Here's how the part is built. I have some questions about the finished solid (model axes, mm). Coordinates: 2 decimals unless noted, no trailing zeros. Write each loop counter-clockwise with the first axis right and the second up, starting at its lowest first coordinate (ties: lowest second). Pieces come first, ordered by that corner, then holes. Notation, with made-up numbers: (-26, -4) - (-19, -4) arc R31 cw to (-19, 30) - close; hole circle Ø8 at (55, -2.75). An arc over 180 degrees is marked (long way). Answer in a Markdown table with one row per item. Add a question column.
Item 1: Imagine slicing it at C-C (x = -20). Please give me the cut outline in (y, z).
Item 2: Imagine slicing it at A-A (y = -22.2). Please give me the cut outline in (x, z), plus the area to 3 significant figures.
Item 3: If I drill on probe 1 along Y at (x, z) = (-20, -6); probe 2 along X at (y, z) = (22.2, -6.25); probe 3 along Y at (x, z) = (-13, -1.75), over which ranges is the centre line in solid material (lowest first)? Write a range as from..to.
Item 4: Imagine slicing it at D-D (z = -9). Please give me the cut outline in (x, y).
Item 5: Imagine slicing it at B-B (x = 13). Please give me the cut outline in (y, z), plus the area to 3 significant figures.
Item 6: I'm going to push a flat-ended pin straight in: pin 1 (4 mm diameter, centred on x = 13, y = 0, fed in from -Z). Where does the tip first touch, or does it pass through?
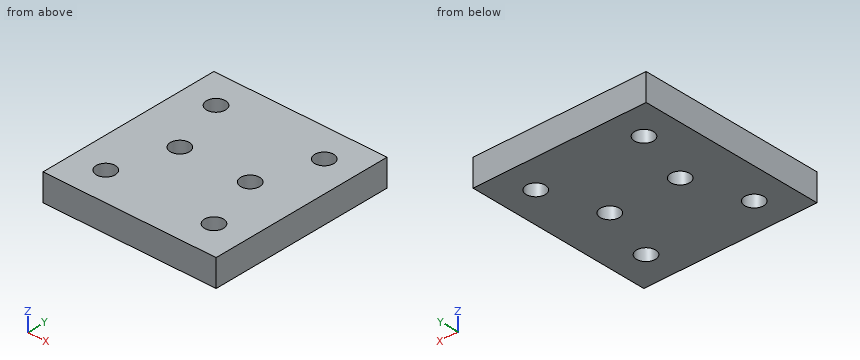
Solid Edge part; units mm, degrees
sketch "Sketch1" plane through (0, 0, 0) normal (0, 0, 1) x (1, 0, 0)
  line L0 (32, -10) -> (32, 10)
  line L1 (32, 10) -> (32, 34.4)
  line L2 (32, 34.4) -> (-32, 34.4)
  line L3 (-32, 34.4) -> (-32, 10)
  line L4 (-32, 10) -> (-32, -10)
  line L5 (-32, -10) -> (-32, -34.4)
  line L6 (-32, -34.4) -> (32, -34.4)
  line L7 (32, -34.4) -> (32, -10)
extrude "Protrusion1" add sketch "Sketch1" against normal blind 10
hole "Hole_1" at (20, -22.2, 0) direction (0, 0, -1) diameter 7 end up to next
mirror "Mirror1" about plane through (0, 0, 0) normal (1, 0, 0) of "Hole_1"
mirror "Mirror2" about plane through (0, 0, 0) normal (0, -1, 0) of "Mirror1", "Hole_1"
hole "Hole_4" at (13, 0, 0) direction (0, 0, -1) diameter 7 end up to next
hole "Hole2" at (-13, 0, 0) direction (0, 0, -1) diameter 7 end up to next
Here are the results:
| question | item | result |
|---|---|---|
| 1 | outline | (-34.4, -10) - (-25.7, -10) - (-25.7, 0) - (-34.4, 0) - close; (-18.7, -10) - (18.7, -10) - (18.7, 0) - (-18.7, 0) - close; (25.7, -10) - (34.4, -10) - (34.4, 0) - (25.7, 0) - close |
| 2 | outline | (-32, -10) - (-23.5, -10) - (-23.5, 0) - (-32, 0) - close; (-16.5, -10) - (16.5, -10) - (16.5, 0) - (-16.5, 0) - close; (23.5, -10) - (32, -10) - (32, 0) - (23.5, 0) - close |
| 2 | area | 500 mm2 |
| 3 | probe 1 | y = -34.4..-25.7, -18.7..18.7, 25.7..34.4 |
| 3 | probe 2 | x = -32..-23.5, -16.5..16.5, 23.5..32 |
| 3 | probe 3 | y = -34.4..-3.5, 3.5..34.4 |
| 4 | outline | (-32, -34.4) - (32, -34.4) - (32, 34.4) - (-32, 34.4) - close; hole circle Ø7 at (-20, -22.2); hole circle Ø7 at (-20, 22.2); hole circle Ø7 at (-13, 0); hole circle Ø7 at (13, 0); hole circle Ø7 at (20, -22.2); hole circle Ø7 at (20, 22.2) |
| 5 | outline | (-34.4, -10) - (-3.5, -10) - (-3.5, 0) - (-34.4, 0) - close; (3.5, -10) - (34.4, -10) - (34.4, 0) - (3.5, 0) - close |
| 5 | area | 618 mm2 |
| 6 | pin 1 | passes through |
